Check sheet for the modelled part. Datum: model origin and axes. Units: mm. Face numbers are marked on the shaded views. A direction names the side the tool comes from. Give positions to 0.01 mm unless a question says otherwise; leave off trailing zeros. Order: outer loops, then holes, each group sorted by start corner. A loop starts at its lowest first (then second) coordinate and runs counter-clockwise, first axis right, second up.
Item 1: Sectioned sample at B-B on x = 20.5. Record the boundary of the cut face in (y, z).
Item 2: Gauge pin test, flat ends, axial feed: P1, Ø4, axis at y = 20, z = 24, coming from the +X side; P2, Ø1.8, axis at y = 20, z = -24, coming from the +X side; P3, Ø10, axis at y = 35.5, z = 10.5, coming from the +X side; P4, Ø2, axis at x = -12, z = -9.5, coming from the +Y side. Record the tip position at first contact, or that the pin passes through.
Item 3: Access from +Z, -Z, +X, -X, +Y, -Y to the whole of each face (thin tool, end or side, straight path). Record for the marked faces 5 and 6.
Item 4: Sectioned sample at A-A on y = 26.5. Record the boundary of the cut face in (x, z), and give its area (3 significant figures).
Item 5: Release check for a two-part mould opening along Z. For the marked faces 1, 2, 3 and 4 record: released by +Z, released by -Z, zero draft, split by the parting line, or undercut.
Item 6: Material ranges on line 1 along Y through (x, z) = (36.4, 24); line 2 along Z through (x, y) = (-30, 31); line 3 along Y through (x, z) = (-11, -24), recorded low to high.
Item 7: Sectioned sample at D-D on z = -11. Record the boundary of the cut face in (x, y).
Item 8: Sectioned sample at C-C on y = 5.5. Record the boundary of the cut face in (x, z), and give its area (3 significant figures).
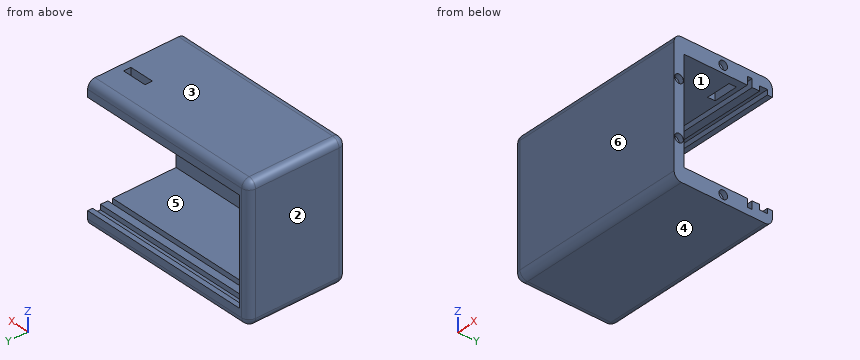
from build123d import *

# Parameters (mm, degrees)
ESQUISSE1_W             = 75
ESQUISSE1_H             = 54
BOSS_EXTRU_1_DEPTH      = 40
ESQUISSE2_W             = 42
ESQUISSE2_H             = 36.230264554
ENL_V_MAT_EXTRU_1_DEPTH = 71
ESQUISSE4_W             = 2
ESQUISSE4_H             = 3.2
ESQUISSE4_W_2           = 3.3
ESQUISSE4_H_2           = 2
ENL_V_MAT_EXTRU_2_DEPTH = 72
ESQUISSE8_W             = 10
ESQUISSE8_H             = 3
ENL_V_MAT_EXTRU_5_DEPTH = 11
ESQUISSE9_R             = 1.75
ENL_V_MAT_EXTRU_6_DEPTH = 2
CONG_1_R                = 3


with BuildPart() as part:
    # Esquisse1 → Boss.-Extru.1 (new body)
    with BuildSketch(Plane(origin=(0, 0, 0), x_dir=(1, 0, 0), z_dir=(0, 1, 0))):
        Rectangle(ESQUISSE1_W, ESQUISSE1_H)
    extrude(amount=BOSS_EXTRU_1_DEPTH)

    # Esquisse2 → Enlèv. mat.-Extru.1 (cut)
    with BuildSketch(Plane(origin=(37.5, 0, 0), x_dir=(0, 0, -1), z_dir=(1, 0, 0))):
        with Locations((0, 22.115132277)):
            Rectangle(ESQUISSE2_W, ESQUISSE2_H)
    extrude(amount=-ENL_V_MAT_EXTRU_1_DEPTH, mode=Mode.SUBTRACT)

    # Esquisse4 → Enlèv. mat.-Extru.2 (cut)
    with BuildSketch(Plane(origin=(-33.5, 0, 0), x_dir=(0, 0, -1), z_dir=(1, 0, 0))):
        with Locations((-22, 36.4)):
            Rectangle(ESQUISSE4_W, ESQUISSE4_H)
        with Locations((-22.65, 30.8)):
            Rectangle(ESQUISSE4_W_2, ESQUISSE4_H_2)
        with Locations((22, 36.4)):
            Rectangle(ESQUISSE4_W, ESQUISSE4_H)
        with Locations((22.65, 30.8)):
            Rectangle(ESQUISSE4_W_2, ESQUISSE4_H_2)
    extrude(amount=ENL_V_MAT_EXTRU_2_DEPTH, mode=Mode.SUBTRACT)

    # Esquisse8 → Enlèv. mat.-Extru.5 (cut)
    with BuildSketch(Plane.XY.offset(27)):
        with Locations((29.5, 26.5)):
            Rectangle(ESQUISSE8_W, ESQUISSE8_H)
    extrude(amount=-ENL_V_MAT_EXTRU_5_DEPTH, mode=Mode.SUBTRACT)

    # Esquisse9 → Enlèv. mat.-Extru.6 (cut)
    with BuildSketch(Plane(origin=(37.5, 0, 0), x_dir=(0, 0, -1), z_dir=(1, 0, 0))):
        with Locations((-24, 20)):
            Circle(ESQUISSE9_R)
        with Locations((-11, 2)):
            Circle(ESQUISSE9_R)
        with Locations((11, 2)):
            Circle(ESQUISSE9_R)
        with Locations((24, 20)):
            Circle(ESQUISSE9_R)
    extrude(amount=-ENL_V_MAT_EXTRU_6_DEPTH, mode=Mode.SUBTRACT)

    # Congé1
    cong_1_edges = [part.edges().sort_by_distance(p)[0] for p in [
        (-37.5, 40, 0),
        (0, 40, 27),
        (0, 0, 27),
        (-37.5, 0, 0),
        (0, 0, -27),
        (-37.5, 20, 27),
        (-37.5, 20, -27),
        (0, 40, -27),
    ]]
    fillet(cong_1_edges, radius=CONG_1_R)


solid = part.part
Report:
1. outline: (0, -24) arc R3 ccw to (3, -27) - (37, -27) arc R3 ccw to (40, -24) - (40, -21) - (38, -21) - (38, -23) - (34.8, -23) - (34.8, -21) - (31.8, -21) - (31.8, -24.3) - (29.8, -24.3) - (29.8, -21) - (4, -21) - (4, 21) - (29.8, 21) - (29.8, 24.3) - (31.8, 24.3) - (31.8, 21) - (34.8, 21) - (34.8, 23) - (38, 23) - (38, 21) - (40, 21) - (40, 24) arc R3 ccw to (37, 27) - (3, 27) arc R3 ccw to (0, 24) - close
2. P1: stops at x = 37.5
2. P2: stops at x = 35.5
2. P3: stops at x = -33.5
2. P4: stops at y = 4
3. face 5: +X, +Y
3. face 6: +Z, -Z, +X, -X, -Y
4. outline: (-37.5, -24) arc R3 ccw to (-34.5, -27) - (37.5, -27) - (37.5, -21) - (-33.5, -21) - (-33.5, 21) - (24.5, 21) - (24.5, 27) - (-34.5, 27) arc R3 ccw to (-37.5, 24) - close; (34.5, 21) - (37.5, 21) - (37.5, 27) - (34.5, 27) - close
4. area: 1,000 mm2
5. face 1: undercut
5. face 2: zero draft
5. face 3: released by +Z
5. face 4: released by -Z
6. line 1: y = 0 to 18.25, 21.75 to 29.8, 31.8 to 40
6. line 2: z = -27 to -24.3, 24.3 to 27
6. line 3: y = 0 to 29.8, 31.8 to 40
7. outline: (-37.5, 3) arc R3 ccw to (-34.5, 0) - (37.5, 0) - (37.5, 0.25) - (35.5, 0.25) - (35.5, 3.75) - (37.5, 3.75) - (37.5, 4) - (-33.5, 4) - (-33.5, 40) - (-34.5, 40) arc R3 ccw to (-37.5, 37) - close
8. outline: (-37.5, -24) arc R3 ccw to (-34.5, -27) - (37.5, -27) - (37.5, -21) - (-33.5, -21) - (-33.5, 21) - (37.5, 21) - (37.5, 27) - (-34.5, 27) arc R3 ccw to (-37.5, 24) - close
8. area: 1,060 mm2
